Autodesk Inventor part; units mm, degrees
ref_plane "Work Plane1" through (5.485, 0.042, -3) normal (0, 0, -1) x (0, 1, 0)
ref_plane "YZ Plane" through (0, 0, 0) normal (1, 0, 0) x (0, 1, 0)
ref_plane "XZ Plane" through (0, 0, 0) normal (0, 1, 0) x (-1, 0, 0)
sketch "Sketch1" plane through (0, 0, 0) normal (0, 0, 1) x (1, 0, 0)
  line L0 (7.011, 4.2884) -> (7.2242, 4.5036)
  line L1 (9.7459, 1.5804) -> (9.5018, 1.4012)
  line L2 (10.4101, 2.9001) -> (10.3642, 2.6007)
  line L3 (6.7053, 2.2945) -> (6.6103, 2.5821)
  line L4 (9.2149, 4.8291) -> (9.4855, 4.6929)
  circle A0 centre (8.485, 3.042) radius 1
  circle A1 centre (8.485, 3.042) radius 1.9244
  circle A2 centre (0, 0) radius 4.2028
  circle A3 centre (0, 0) radius 1
extrude "Extrusion1" add sketch "Sketch1" against normal blind 1 contours A2
sketch "Sketch2" plane through (0, 0, -1) normal (0, 0, -1) x (-1, 0, 0)
  circle A0 centre (0, 0) radius 4.2028
  circle A1 centre (0, 0) radius 1
  line L0 (-6.5615, 2.8811) -> (-6.56, 3.184)
  line L1 (-9.4855, 4.6929) -> (-9.7314, 4.516)
  line L2 (-8.945, 1.1673) -> (-8.646, 1.1184)
  circle A2 centre (-8.485, 3.042) radius 1
  circle A3 centre (-8.485, 3.042) radius 1.9485
  circle A4 centre (0, 0) radius 3.5115
extrude "Extrusion2" add sketch "Sketch2" along normal blind 1 contours A4
sketch "Sketch3" plane through (0, 0, -2) normal (0, 0, -1) x (-1, 0, 0)
  circle A0 centre (0, 0) radius 4.2028
  circle A1 centre (0, 0) radius 1
  circle A2 centre (0, 0) radius 1
ref_plane "Work Plane1" through (5.485, 0.042, -3) normal (0, 0, -1) x (0, 1, 0)
extrude "Extrusion3" add sketch "Sketch3" along normal up to surface (1 mm away)
chamfer "Chamfer1" distance 0.6 angle 45 2 edges at (4.2028, 0, -2) (-4.2028, 0, -1)
properties part number "koło_pasowe_duze"
Source: CAD feature listing. Evaluate the final solid. Frame: model axes, mm. Give positions to 0.01 mm unless a question says otherwise; leave off trailing zeros. Write each loop counter-clockwise with the first axis right and the second up, starting at its lowest first coordinate (ties: lowest second). Pieces come first, ordered by that corner, then holes. Notation, with made-up numbers: M 58.25,71.5 L 99.25,71.5 A25 ccw 99.25,98.5 Z; hole C 40.5,-33 d6. An arc over 180 degrees is marked long. Return JSON: item names as keys, results as strings. Group by question number.
1) Ray query, L1, parallel to Y at x = 0, z = -1.65; L2, parallel to X at y = 0.25, z = -1.8; L3, parallel to Z at x = 2.25, y = 3. Return the intervals inside material, ascending.
2) Cut plane A-A, the plane x = 0. Output: boundary loops of the cut face in (y, z), then the cut area to 3 significant figures.
3) First-contact query: pin 1 Ø1.6 at (x, y) = (0, 0) entering from +Z; pin 2 Ø1 at (x, z) = (1.5, -0.5) entering from +Y. Flat tips, straight axial feed; report the tip coordinate or a pass-through.
4) Draft query along Z for faces 1 (the face through (-1.62, 3.115, -1.493)), 2 (the face through (1, -1, 0)), 3 (the face through (-1, -1, -3)), 4 (the face through (-4.01, -1.26, -2.8)). Return one class per face: released by +Z, released by -Z, zero draft, split by the parting line, or undercut.
Data:
{
 "1": {"L1": "y = -3.51 to -1, 1 to 3.51", "L2": "x = -3.5 to -0.97, 0.97 to 3.5", "L3": "z = -3 to -2.15, -0.85 to 0"},
 "2": {"outline": "M -4.2,-3 L -1,-3 L -1,0 L -4.2,0 L -4.2,-0.4 L -3.6,-1 L -3.51,-1 L -3.51,-2 L -3.6,-2 L -4.2,-2.6 Z; M 1,-3 L 4.2,-3 L 4.2,-2.6 L 3.6,-2 L 3.51,-2 L 3.51,-1 L 3.6,-1 L 4.2,-0.4 L 4.2,0 L 1,0 Z", "area": "17.1 mm²"},
 "3": {"pin 1": "passes through", "pin 2": "stops at y = 4.08"},
 "4": {"face 1": "undercut", "face 2": "released by +Z", "face 3": "released by -Z", "face 4": "zero draft"}
}
